Can you work these out from the model? Positions are in its coordinate system, mm. Face numbers are marked on the shaded views. A direction names the side the tool comes from. Round coordinates to 2 decimals unless told otherwise and drop trailing zeros. Order: outer loops, then holes, each group sorted by start corner. A loop starts at its lowest first (then second) coordinate and runs counter-clockwise, first axis right, second up. Notation, with made-up numbers: (-28, 59.25) -> (16, 59.25) arc R23 cw to (16, 82.25) -> close; hole circle Ø10 at (81, 50.5). An arc over 180 degrees is marked (long way). One line per item, written item: value.
```python
from build123d import *

# Parameters (mm, degrees)
SALIENTE_EXTRUIR1_DEPTH      = 6.5024
SALIENTE_EXTRUIR1_DEPTH_BACK = 6.5024
SALIENTE_EXTRUIR2_DEPTH      = 5.0038
SALIENTE_EXTRUIR2_DEPTH_BACK = 5.0038
CROQUIS1_4_W                 = 5.9944
CROQUIS1_4_H                 = 3.9878
SALIENTE_EXTRUIR3_DEPTH      = 3.4671
SALIENTE_EXTRUIR3_DEPTH_BACK = 3.4671
CROQUIS2_W                   = 5.0038
CROQUIS2_H                   = 0.508
CROQUIS2_H_2                 = 1.524
CROQUIS2_W_2                 = 1.4986
CROQUIS2_H_3                 = 10.4902
CORTAR_EXTRUIR1_DEPTH        = 0.508
CROQUIS3_OUTSIDE_W           = 20.026
CROQUIS3_OUTSIDE_H           = 23.024
CORTAR_EXTRUIR2_DEPTH        = 3.9878


with BuildPart() as part:
    # Croquis1 → Saliente-Extruir1 (new body, two sides)
    with BuildSketch(Plane(origin=(0, 0, 0), x_dir=(0, 0, -1), z_dir=(1, 0, 0))) as saliente_extruir1_sk:
        Polygon((-3.5052, 3.0099), (-7.493, 3.0099), (-8.001, 3.0099), (-8.001, 2.5019), (-7.0104, 2.5019), (-7.0104, -2.5019), (7.0104, -2.5019), (7.0104, 2.5019), (8.001, 2.5019), (8.001, 3.0099), (6.477, 3.0099), align=None)
    extrude(amount=SALIENTE_EXTRUIR1_DEPTH)
    extrude(saliente_extruir1_sk.sketch, amount=-SALIENTE_EXTRUIR1_DEPTH_BACK)

    # Croquis1<3> → Saliente-Extruir2 (add, two sides)
    with BuildSketch(Plane(origin=(0, 0, 0), x_dir=(0, 0, -1), z_dir=(1, 0, 0))) as saliente_extruir2_sk:
        with BuildLine():
            Line((-2.868527833, 7.8359), (-3.376527833, 7.8359))
            Line((-3.376527833, 7.8359), (-7.493, 3.0099))
            Line((-7.493, 3.0099), (-3.5052, 3.0099))
            Line((-3.5052, 3.0099), (6.477, 3.0099))
            Line((6.477, 3.0099), (4.937272491, 7.021027296))
            ThreePointArc((4.937272491, 7.021027296), (4.47096127, 7.61254026), (3.751625349, 7.8359))
            Line((3.751625349, 7.8359), (3.125872167, 7.8359))
            Line((3.125872167, 7.8359), (-2.868527833, 7.8359))
        make_face()
    extrude(amount=SALIENTE_EXTRUIR2_DEPTH)
    extrude(saliente_extruir2_sk.sketch, amount=-SALIENTE_EXTRUIR2_DEPTH_BACK)

    # Croquis1<4> → Saliente-Extruir3 (add, two sides)
    with BuildSketch(Plane(origin=(0, 0, 0), x_dir=(0, 0, -1), z_dir=(1, 0, 0))) as saliente_extruir3_sk:
        with Locations((0.128672167, 9.8298)):
            Rectangle(CROQUIS1_4_W, CROQUIS1_4_H)
    extrude(amount=SALIENTE_EXTRUIR3_DEPTH)
    extrude(saliente_extruir3_sk.sketch, amount=-SALIENTE_EXTRUIR3_DEPTH_BACK)

    # Croquis2 → Cortar-Extruir1 (cut)
    with BuildSketch(Plane(origin=(0, 3.0099, 0), x_dir=(1, 0, 0), z_dir=(0, 1, 0))):
        with Locations((0, -7.747)):
            Rectangle(CROQUIS2_W, CROQUIS2_H)
        with Locations((0, 7.239)):
            Rectangle(CROQUIS2_W, CROQUIS2_H_2)
        with Locations((-5.7531, 0)):
            Rectangle(CROQUIS2_W_2, CROQUIS2_H_3)
        with Locations((5.7531, 0)):
            Rectangle(CROQUIS2_W_2, CROQUIS2_H_3)
    extrude(amount=-CORTAR_EXTRUIR1_DEPTH, mode=Mode.SUBTRACT)

    # Croquis3 outside → Cortar-Extruir2 (cut)
    with BuildSketch(Plane(origin=(0, 11.8237, 0), x_dir=(1, 0, 0), z_dir=(0, 1, 0))):
        Rectangle(CROQUIS3_OUTSIDE_W, CROQUIS3_OUTSIDE_H)
        Polygon((-3.4671, 3.125872167), (-3.4671, -2.868527833), (-1.9685, -2.868527833), (-1.9685, -2.614527833), (-3.2131, -2.614527833), (-3.2131, 2.871872167), (-1.9685, 2.871872167), (-1.9685, 3.125872167), align=None, mode=Mode.SUBTRACT)
        Polygon((0.508, 1.9685), (-0.508, 1.9685), (-0.508, 0.508), (-1.9685, 0.508), (-1.9685, -0.508), (-0.508, -0.508), (-0.508, -1.9685), (0.508, -1.9685), (0.508, -0.508), (1.9685, -0.508), (1.9685, 0.508), (0.508, 0.508), align=None, mode=Mode.SUBTRACT)
        Polygon((3.2131, 2.871872167), (3.2131, -2.614527833), (1.9685, -2.614527833), (1.9685, -2.868527833), (3.4671, -2.868527833), (3.4671, 3.125872167), (1.9685, 3.125872167), (1.9685, 2.871872167), align=None, mode=Mode.SUBTRACT)
    extrude(amount=-CORTAR_EXTRUIR2_DEPTH, mode=Mode.SUBTRACT)


solid = part.part
```
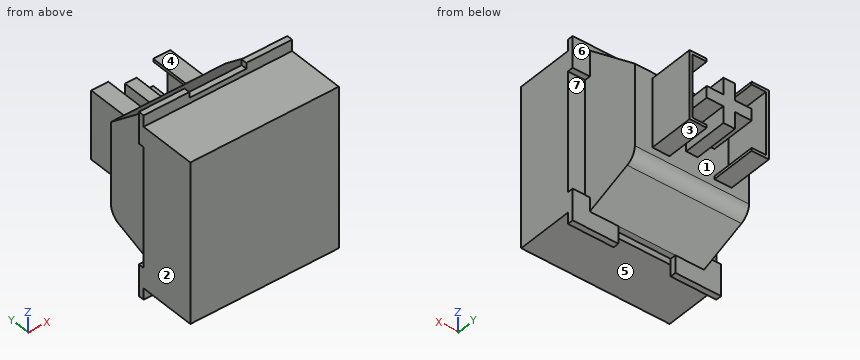
Q1. On a 3-axis mill with a long thin cutter (end or side, diameter ignored), from which of +Z, -Z, +X, -X, +Y, -Y can I reach the whole of each face in a straight line? I mean the marked faces 4, 5, 6 and 7. Say none if no direction works.
Answers below:
face 4: +Z, +X, -X, +Y
face 5: -Z, +X, -X, -Y
face 6: +Z, +X, +Y
face 7: +X, +Y
Q2. I want a section at C-C on z = -4.5. List the corners of the cut face in (x, y) for me.
Answers below:
outline: (-6.5, -2.5) -> (6.5, -2.5) -> (6.5, 2.5) -> (5, 2.5) -> (5, 7.59) -> (-5, 7.59) -> (-5, 2.5) -> (-6.5, 2.5) -> close
Q3. We'd pull the mould along X, two halves only. Please class the marked faces 1, 2 and 3: released by +X, released by -X, zero draft, split by the parting line, or undercut.
Answers below:
face 1: undercut
face 2: released by -X
face 3: zero draft
Q4. Will these pins go through, and if not, where does the flat tip stop? pin 1 Ø1.5 at (x, y) = (1, 0.5) entering from +Z; pin 2 Ø2 at (y, z) = (4.5, -6.5) entering from -X; pin 3 Ø2.5 at (x, y) = (2, 1) entering from -Z.
Answers below:
pin 1: z = 7.01
pin 2: x = -5
pin 3: z = -7.01
Q5. I want a section at B-B on x = 5.5. List the corners of the cut face in (y, z) for me.
Answers below:
outline: (-2.5, -7.01) -> (2.5, -7.01) -> (2.5, -8) -> (3.01, -8) -> (3.01, -5.25) -> (2.5, -5.25) -> (2.5, 5.25) -> (3.01, 5.25) -> (3.01, 8) -> (2.5, 8) -> (2.5, 7.01) -> (-2.5, 7.01) -> close
Q6. Please list where these lines run through material, in increasing order: line 1 along X through (y, z) = (11.25, 1); line 2 along X through (y, z) = (11, -0.25); line 3 along X through (y, z) = (6.5, -4.25).
Answers below:
line 1: -3.47 to -3.21, -0.51 to 0.51, 3.21 to 3.47
line 2: -3.47 to -3.21, -1.97 to 1.97, 3.21 to 3.47
line 3: -5 to 5
Q7. I want a section at A-A on y = 8.5. List the corners of the cut face in (x, z) for me, plus the area to 3 significant figures.
Answers below:
outline: (-3.47, -3.13) -> (-1.97, -3.13) -> (-1.97, -2.87) -> (-3.21, -2.87) -> (-3.21, 2.61) -> (-1.97, 2.61) -> (-1.97, 2.87) -> (-3.47, 2.87) -> close; (-1.97, -0.51) -> (-0.51, -0.51) -> (-0.51, -1.97) -> (0.51, -1.97) -> (0.51, -0.51) -> (1.97, -0.51) -> (1.97, 0.51) -> (0.51, 0.51) -> (0.51, 1.97) -> (-0.51, 1.97) -> (-0.51, 0.51) -> (-1.97, 0.51) -> close; (1.97, -3.13) -> (3.47, -3.13) -> (3.47, 2.87) -> (1.97, 2.87) -> (1.97, 2.61) -> (3.21, 2.61) -> (3.21, -2.87) -> (1.97, -2.87) -> close
area: 11.3 mm^2
Q8. I want a section at D-D on x = 4. List the corners of the cut face in (y, z) for me.
Answers below:
outline: (-2.5, -7.01) -> (2.5, -7.01) -> (2.5, -8) -> (3.01, -8) -> (3.01, -6.48) -> (7.02, -4.94) arc R1.27 ccw to (7.84, -3.75) -> (7.84, 3.38) -> (3.01, 7.49) -> (3.01, 8) -> (2.5, 8) -> (2.5, 7.01) -> (-2.5, 7.01) -> close
